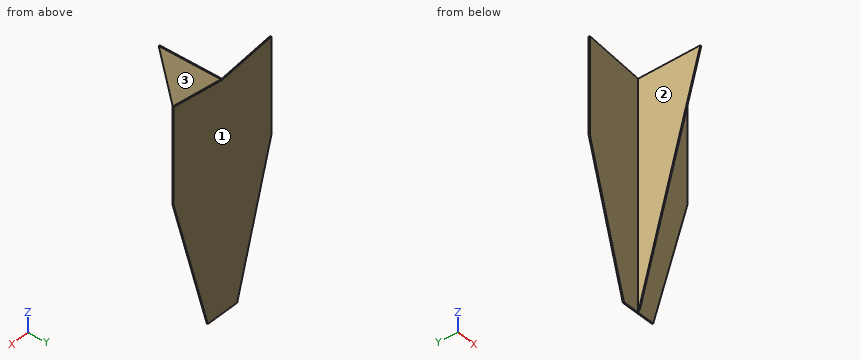
```python
from build123d import *

# Parameters (mm, degrees)
SKETCH_1_W           = 100
SKETCH_1_H           = 210
EXTRUDE_1_DEPTH      = 1
CUT_EXTRUDE_1_DEPTH  = 1
EXTRUDE_2_DEPTH      = 0.5
EXTRUDE_2_DEPTH_BACK = 0.5


with BuildPart() as part:
    # ｽｹｯﾁ1 → ﾎﾞｽ - 押し出し1 (new body)
    with BuildSketch(Plane(origin=(0, 0, 0), x_dir=(1, 0, 0), z_dir=(0, 1, 0))):
        Rectangle(SKETCH_1_W, SKETCH_1_H)
    extrude(amount=EXTRUDE_1_DEPTH)

    # ｽｹｯﾁ2 → ｶｯﾄ - 押し出し1 (cut)
    with BuildSketch(Plane(origin=(0, 1, 0), x_dir=(1, 0, 0), z_dir=(0, 1, 0))):
        Polygon((15, 105), (50, -17.5), (50, 105), align=None)
        Polygon((-50, 105), (-50, -17.5), (-15, 105), align=None)
        Polygon((50, -105), (50, -101.666666667), (0, -95), (-50, -101.666666667), (-50, -105), align=None)
    extrude(amount=-CUT_EXTRUDE_1_DEPTH, mode=Mode.SUBTRACT)

    # ｽｹｯﾁ4 → ﾎﾞｽ - 押し出し2 (add, two sides: drawn at the far end of the back side and taken through both)
    with BuildSketch(Plane(origin=(0, 0, 0), x_dir=(0, 0, -1), z_dir=(1, 0, 0)).offset(-EXTRUDE_2_DEPTH_BACK)):
        Polygon((105, 0), (-95, -55), (-95, 0), align=None)
    extrude(amount=EXTRUDE_2_DEPTH + EXTRUDE_2_DEPTH_BACK)


solid = part.part
```
Input: part model. Units: mm. Frame: model coordinates. Face numbers are marked on the shaded views. A direction names the side the tool comes from. Coordinates: 2 decimals unless noted, no trailing zeros. Loops run counter-clockwise (first coordinate to the right, second up) from the corner with the lowest first, then second, coordinate; pieces in that order, holes last. Notation, with made-up numbers: M -9,44 L 34,44 A34 ccw 34,80 Z; hole C 16.25,86 d1. An arc over 180 degrees is marked long. Use a Markdown table: item, result. Add a question column.
1) Section A-A, the plane z = 61. Return the cut outline in (x, y), plus the area to 3 significant figures.
2) Line query: L1, parallel to Y at x = -33.5, z = 1.5; L2, parallel to X at y = -6, z = -40. Output: solid intervals per line, ascending. Write a range as from..to.
3) Set-up query: the marked faces 1, 2 and 3. Return all of +Z, -Z, +X, -X, +Y, -Y with unobstructed straight access to the full face (end or side cutting, diameter ignored); none if empty.
4) Section D-D, the plane z = -10.5. Return the cut outline in (x, y).
5) Pin query (flat end, axial travel): P1, Ø2, axis at x = -18.5, z = -68, coming from the -Y side; P2, Ø5, axis at y = -9, z = 68, coming from the +X side; P3, Ø1, axis at y = -24, z = 65, coming from the -X side. Return the tip coordinate at first contact, or that it passes through.
6) Section B-B, the plane x = -31.5. Return the cut outline in (y, z).
7) Section C-C, the plane y = -40. Return the cut outline in (x, z), plus the area to 3 significant figures.
Answer below:
| question | item | result |
|---|---|---|
| 1 | outline | M -50,0 L -0.5,0 L -0.5,-45.65 L 0.5,-45.65 L 0.5,0 L 50,0 L 50,1 L -50,1 Z |
| 1 | area | 146 mm2 |
| 2 | L1 | 0..1 |
| 2 | L2 | -0.5..0.5 |
| 3 | face 1 | +Z, -Z, +X, -X, +Y |
| 3 | face 2 | +Z, -Z, -X, -Y |
| 3 | face 3 | +Z, -Z, +X, -Y |
| 4 | outline | M -42,0 L -0.5,0 L -0.5,-25.99 L 0.5,-25.99 L 0.5,0 L 42,0 L 42,1 L -42,1 Z |
| 5 | P1 | y = 0 |
| 5 | P2 | x = 0.5 |
| 5 | P3 | x = -0.5 |
| 6 | outline | M 0,-47.25 L 1,-47.25 L 1,99.2 L 0,99.2 Z |
| 7 | outline | M -0.5,40.45 L 0.5,40.45 L 0.5,95 L -0.5,95 Z |
| 7 | area | 54.5 mm2 |
